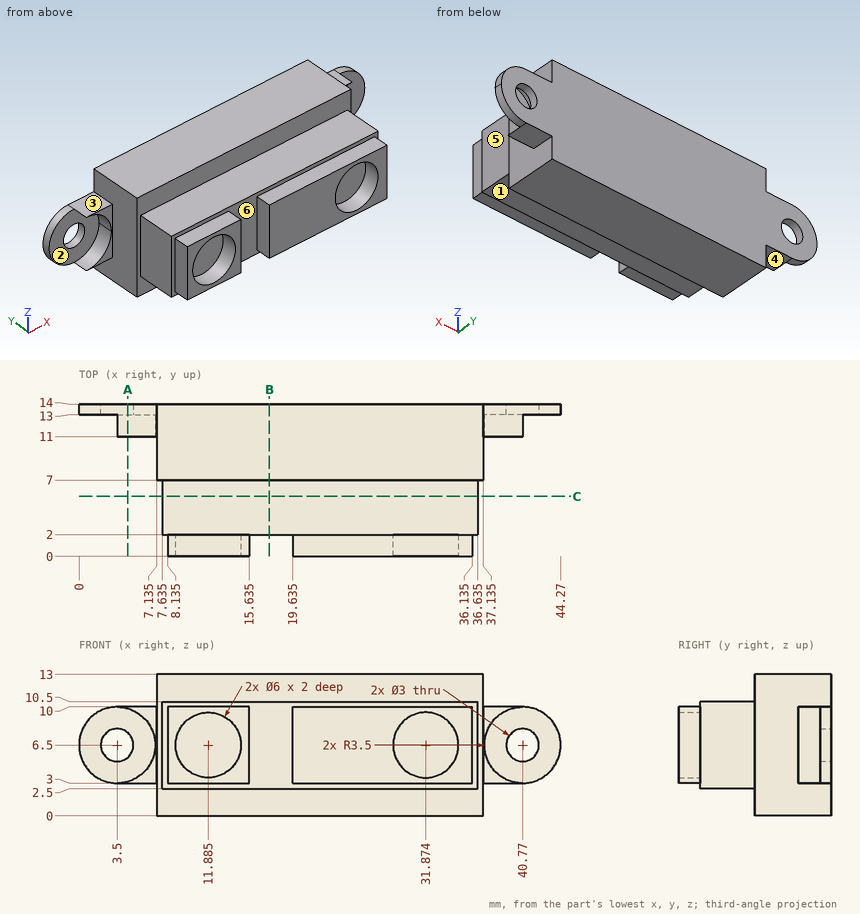
Check sheet for the drawn part. Datum: minimum x, y, z corner. Units: mm. A direction names the side the tool comes from. Round coordinates to 2 decimals unless told otherwise and drop trailing zeros. Write each loop counter-clockwise with the first axis right and the second up, starting at its lowest first coordinate (ties: lowest second). Pieces come first, ordered by that corner, then holes. Notation, with made-up numbers: (57.5, -7.5) - (103.5, -7.5) arc R18 cw to (103.5, 14.5) - close; hole circle Ø10 at (-18, -10.5). An arc over 180 degrees is marked (long way). Write each question's results on one line, items separated by ' | '.
(1) Thickness scan on probe 1 along Z at (x, y) = (3.5, 13.35); probe 2 along Y at (x, z) = (36.5, 4); probe 3 along Z at (x, y) = (31.5, 5). Record the ranges inside material, lowest first. Write a range as from..to.
Computed:
probe 1: z = 3..5, 8..10 | probe 2: y = 2..14 | probe 3: z = 2.5..10.5
(2) Draft check along X on the marked faces 4, 5 and 6. Enter one of: pulls with the +X half, pulls with the -X half, needs draft (parallel to the pull), parting line crosses it, or undercut.
Computed:
face 4: needs draft | face 5: pulls with the +X half | face 6: undercut
(3) Sectioned sample at B-B, the plane x = 17.5. Enter the section's corners in (y, z).
Computed:
outline: (2, 2.5) - (7, 2.5) - (7, 0) - (14, 0) - (14, 13) - (7, 13) - (7, 10.5) - (2, 10.5) - close
(4) Set-up check for the marked faces 1, 2 and 3: record each of +Z, -Z, +X, -X, +Y, -Y from which the full face is reachable in a straight line by a thin tool's end or side.
Computed:
face 1: -Z, +X, -X, -Y | face 2: -X, -Y | face 3: +Z, -X, +Y, -Y
(5) Sectioned sample at C-C, the plane y = 5.5. Enter the section's corners in (x, z) (3 decimals).
Computed:
outline: (7.635, 2.5) - (36.635, 2.5) - (36.635, 10.5) - (7.635, 10.5) - close
(6) Depth check by flat-ended pin: pin 1 Ø5 at (y, z) = (11.5, 9) entering from -X; pin 2 Ø2 at (x, z) = (39, 5.5) entering from -Y; pin 3 Ø1.6 at (x, y) = (27.5, 0.5) entering from -Z; pin 4 Ø2 at (x, y) = (38.5, 7.5) entering from -Z. Enter the tip coordinate at first touch or a pass-through.
Computed:
pin 1: stops at x = 0.04 | pin 2: stops at y = 13 | pin 3: stops at z = 3 | pin 4: passes through
(7) Sectioned sample at A-A, the plane x = 4.5. Enter the section's corners in (y, z).
Computed:
outline: (11, 3) - (14, 3) - (14, 5.38) - (13, 5.38) - (13, 3.15) - (11, 3.15) - close; (11, 9.85) - (13, 9.85) - (13, 7.62) - (14, 7.62) - (14, 10) - (11, 10) - close
